Autodesk Inventor part; units mm, degrees
ref_plane "YZ Plane" through (0, 0, 0) normal (1, 0, 0) x (0, 1, 0)
ref_plane "XZ Plane" through (0, 0, 0) normal (0, 1, 0) x (-1, 0, 0)
ref_plane "XY Plane" through (0, 0, 0) normal (0, 0, 1) x (1, 0, 0)
sketch "Sketch1" plane through (0, 0, 0) normal (0, 1, 0) x (-1, 0, 0)
  line L0 (199.9677, 280.6608) -> (-123.8823, 280.6608)
  line L1 (-123.8823, 280.6608) -> (-123.8823, 287.0108)
  line L2 (-123.8823, 287.0108) -> (206.3177, 287.0108)
  line L3 (206.3177, 287.0108) -> (206.3177, -195.5892)
  line L4 (206.3177, -195.5892) -> (-123.8823, -195.5892)
  line L5 (-123.8823, -195.5892) -> (-123.8823, -189.2392)
  line L6 (-123.8823, -189.2392) -> (199.9677, -189.2392)
  line L7 (199.9677, -189.2392) -> (199.9677, 280.6608)
  point P0 (0, 0)
  dimension "d0" = 482.6
  dimension "d1" = 330.2
  dimension "d2" = 6.35
  dimension "d3" = 6.35
  dimension "d4" = 6.35
extrude "Extrusion1" add sketch "Sketch1" along normal blind 114.3
fillet "Fillet1" radius 3.175 2 edges at (-206.3177, 57.15, 287.0108) (-206.3177, 57.15, -195.5892)
properties part number "Visor"
Input: part model. Units: mm. Frame: model coordinates. A direction names the side the tool comes from. Give positions to 0.01 mm unless a question says otherwise; leave off trailing zeros. Order: outer loops, then holes, each group sorted by start corner. A loop starts at its lowest first (then second) coordinate and runs counter-clockwise, first axis right, second up.
Q1. Ray query, probe 1 along Z at (x, y) = (-11.5, 15.5); probe 2 along X at (y, z) = (95, -83). Return the intervals inside material, ascending.
Checked values:
probe 1: z = -195.59 to -189.24, 280.66 to 287.01
probe 2: x = -206.32 to -199.97
Q2. Section B-B on y = 67. Output: boundary loops of the cut face in (x, z) (3 decimals).
Checked values:
outline: (-206.318, -192.414) arc R3.175 ccw to (-203.143, -195.589) - (123.882, -195.589) - (123.882, -189.239) - (-199.968, -189.239) - (-199.968, 280.661) - (123.882, 280.661) - (123.882, 287.011) - (-203.143, 287.011) arc R3.175 ccw to (-206.318, 283.836) - close
Q3. Section C-C on z = 128. Output: boundary loops of the cut face in (x, y), and give its area (3 significant figures).
Checked values:
outline: (-206.32, 0) - (-199.97, 0) - (-199.97, 114.3) - (-206.32, 114.3) - close
area: 726 mm2
Q4. Contact query for a flat-ended pin moving along its axis: pin 1 Ø4 at (y, z) = (68, 133) entering from +X. Output: stop coordinate, or through.
Checked values:
pin 1: stops at x = -199.97
Q5. Section A-A on x = -103. Output: boundary loops of the cut face in (y, z), and give its area (3 significant figures).
Checked values:
outline: (0, -195.59) - (114.3, -195.59) - (114.3, -189.24) - (0, -189.24) - close; (0, 280.66) - (114.3, 280.66) - (114.3, 287.01) - (0, 287.01) - close
area: 1,450 mm2
Q6. Set-up query: faces 4 (the flat face through (-37, 56, 287.011)), 5 (the flat face through (-40, 56, 280.661)). Return all of +Z, -Z, +X, -X, +Y, -Y with unobstructed straight access to the full face (end or side cutting, diameter ignored); none if empty.
Checked values:
face 4: +Z, +X, -X, +Y, -Y
face 5: +X, +Y, -Y
Q7. Draft query along Z for faces 1 (the flat face through (-206.318, 56, 49)), 2 (the flat face through (-42, 56, -195.589)), 3 (the flat face through (-199.968, 56, 42)). Return one class per face: +Z half, -Z half, draft (parallel to the pull), parting line (faces both ways), or undercut.
Checked values:
face 1: draft
face 2: -Z half
face 3: undercut
